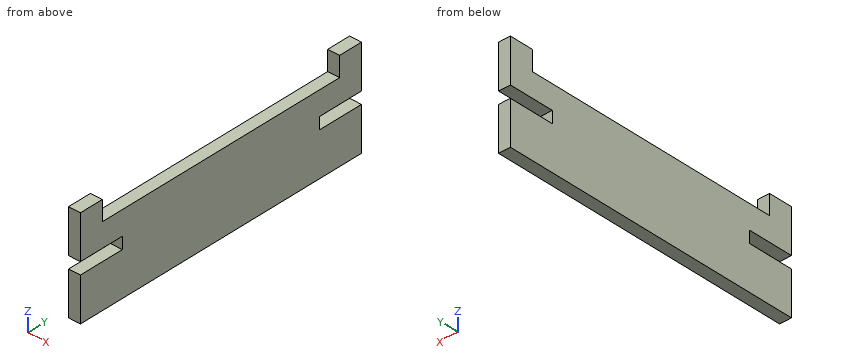
```python
from build123d import *

# Parameters (mm, degrees)
F0_W     = 19.05
F0_H     = 127
F1_DEPTH = 244.871875
F2_W     = 19.05
F2_H     = 38.1
F3_DEPTH = 31.75
F6_DEPTH = 12.7


with BuildPart() as f1:
    # F0 (on Front) → F1 (new body, symmetric)
    with BuildSketch(Plane.XZ):
        Rectangle(F0_W, F0_H)
    extrude(amount=F1_DEPTH, both=True)

    # F2 (on face) → F3 (join)
    with BuildSketch(Plane.XY.offset(63.5)):
        with Locations((0, 225.821875)):
            Rectangle(F2_W, F2_H)
    extrude(amount=F3_DEPTH)

    # F4: F1 across plane


with BuildPart() as f1_1:
    add(f1.part)
    add(f1.part.mirror(Plane.XZ))

    # F5 (on Right) → F6 (cut, symmetric)
    with BuildSketch(Plane.YZ):
        Polygon((-244.871875, 6.35), (-216.296875, 6.35), (-171.846875, 6.35), (-171.846875, 25.4), (-216.296875, 25.4), (-244.871875, 25.4), align=None)
        Polygon((216.296875, 25.4), (171.846875, 25.4), (171.846875, 6.35), (216.296875, 6.35), (244.871875, 6.35), (244.871875, 25.4), align=None)
    extrude(amount=F6_DEPTH, both=True, mode=Mode.SUBTRACT)


solid = f1_1.part
```
Here's how the part is built. I have some questions about the finished solid (model axes, mm). Coordinates: 2 decimals unless noted, no trailing zeros. Loops run counter-clockwise (first coordinate to the right, second up) from the corner with the lowest first, then second, coordinate; pieces in that order, holes last. Notation, with made-up numbers: (72.25, 4.5) - (100.25, 4.5) arc R5 ccw to (100.25, 11.5) - close; hole circle Ø7 at (-17, -25.75). An arc over 180 degrees is marked (long way). Return JSON: item names as keys, results as strings. Group by question number.
Item 1: Will this pin go through, and if not, where does the flat tip stop? P1, Ø5.5, axis at x = -1.5, y = 27, coming from the +Z side.
Item 2: If we section it at A-A on y = 191: Write out the boundary of the cut face in (x, z) (3 decimals).
Item 3: I need wall thicknesses on line 1 (Z direction, x = 4.5, y = -200); line 2 (Y direction, x = -7.5, z = 75); line 3 (Z direction, x = 1.75, y = 91.5). Which ranges of each line are inside material? Lowest first, please. Write a range as from..to.
Item 4: If we section it at B-B on z = 70: Write out the boundary of the cut face in (x, y) (3 decimals), and give its area (3 significant figures).
Item 5: If we section it at C-C on x = -2.5: Write out the boundary of the cut face in (y, z), and give its area (3 significant figures).
Item 6: If we section it at D-D on y = 26: Write out the boundary of the cut face in (x, z) (3 decimals), and give its area (3 significant figures).
Calculated:
{
 "1": {"P1": "stops at z = 63.5"},
 "2": {"outline": "(-9.525, -63.5) - (9.525, -63.5) - (9.525, 6.35) - (-9.525, 6.35) - close; (-9.525, 25.4) - (9.525, 25.4) - (9.525, 63.5) - (-9.525, 63.5) - close"},
 "3": {"line 1": "z = -63.5..6.35, 25.4..63.5", "line 2": "y = -244.87..-206.77, 206.77..244.87", "line 3": "z = -63.5..63.5"},
 "4": {"outline": "(-9.525, -244.872) - (9.525, -244.872) - (9.525, -206.772) - (-9.525, -206.772) - close; (-9.525, 206.772) - (9.525, 206.772) - (9.525, 244.872) - (-9.525, 244.872) - close", "area": "1,450 mm^2"},
 "5": {"outline": "(-244.87, -63.5) - (244.87, -63.5) - (244.87, 6.35) - (171.85, 6.35) - (171.85, 25.4) - (244.87, 25.4) - (244.87, 95.25) - (206.77, 95.25) - (206.77, 63.5) - (-206.77, 63.5) - (-206.77, 95.25) - (-244.87, 95.25) - (-244.87, 25.4) - (-171.85, 25.4) - (-171.85, 6.35) - (-244.87, 6.35) - close", "area": "61,800 mm^2"},
 "6": {"outline": "(-9.525, -63.5) - (9.525, -63.5) - (9.525, 63.5) - (-9.525, 63.5) - close", "area": "2,420 mm^2"}
}
